Can you work these out from the model? Positions are in its coordinate system, mm. A direction names the side the tool comes from. Round coordinates to 2 decimals unless told otherwise and drop trailing zeros. Loops run counter-clockwise (first coordinate to the right, second up) from the corner with the lowest first, then second, coordinate; pieces in that order, holes last. Notation, with made-up numbers: (-11.75, 83) -> (22.25, 83) arc R24 cw to (22.25, 104) -> close; hole circle Ø6 at (-29.75, 7.5). An arc over 180 degrees is marked (long way). Use a Markdown table: item, result.
from build123d import *

# Parameters (mm, degrees)
CYLINDER_R        = 12.5
CYLINDER_DEPTH    = 4
CYLINDER001_R     = 11
CYLINDER001_DEPTH = 4
CYLINDER002_W     = 11
CYLINDER002_H     = 4
CYLINDER002_ANGLE = 66
BOX_W             = 5
BOX_H             = 1.9
BOX_DEPTH         = 4
BOX001_W          = 5
BOX001_H          = 1.9
BOX001_DEPTH      = 4
CYLINDER003_W     = 13
CYLINDER003_H     = 4
CYLINDER003_ANGLE = 60
CYLINDER004_W     = 14.25
CYLINDER004_H     = 4
CYLINDER004_ANGLE = 46
CYLINDER005_W     = 13
CYLINDER005_H     = 4
CYLINDER005_ANGLE = 60
CYLINDER006_W     = 14.25
CYLINDER006_H     = 4
CYLINDER006_ANGLE = 46
FILLET_R          = 0.9
FILLET001_R       = 0.6
FILLET002_R       = 1.2


with BuildPart() as part:
    # Cylinder → Cylinder (join)
    with BuildSketch(Plane.XY):
        Circle(CYLINDER_R)
    extrude(amount=CYLINDER_DEPTH)

    # Cylinder001 → Cylinder001 (cut)
    with BuildSketch(Plane.XY):
        Circle(CYLINDER001_R)
    extrude(amount=CYLINDER001_DEPTH, mode=Mode.SUBTRACT)

    # Cylinder002 → Cylinder002 (revolve, cut)
    with BuildSketch(Plane(origin=(0, 2, 0), x_dir=(0.544639035, 0.8386705679, 0), z_dir=(0.8386705679, -0.544639035, 0))):
        with Locations((5.5, 2)):
            Rectangle(CYLINDER002_W, CYLINDER002_H)
    revolve(axis=Axis((0, 2, 0), (0, 0, 1)), revolution_arc=CYLINDER002_ANGLE, mode=Mode.SUBTRACT)

    # Box → Box (join)
    with BuildSketch(Plane(origin=(5.2, 10, 0), x_dir=(-0.544639035, -0.8386705679, 0), z_dir=(0, 0, 1))):
        with Locations((2.5, 0.95)):
            Rectangle(BOX_W, BOX_H)
    extrude(amount=BOX_DEPTH)

    # Box001 → Box001 (join)
    with BuildSketch(Plane(origin=(-6.811, 9, 0), x_dir=(0.544639035, -0.8386705679, 0), z_dir=(0, 0, 1))):
        with Locations((2.5, 0.95)):
            Rectangle(BOX001_W, BOX001_H)
    extrude(amount=BOX001_DEPTH)

    # Cylinder003 → Cylinder003 (revolve)
    with BuildSketch(Plane(origin=(17.65, -10, 0), x_dir=(-1, 0, 0), z_dir=(0, 1, 0))):
        with Locations((6.5, 2)):
            Rectangle(CYLINDER003_W, CYLINDER003_H)
    revolve(axis=Axis((17.65, -10, 0), (0, 0, 1)), revolution_arc=CYLINDER003_ANGLE)

    # Cylinder004 → Cylinder004 (revolve, cut)
    with BuildSketch(Plane(origin=(21.75, -10, 0), x_dir=(-1, 0, 0), z_dir=(0, 1, 0))):
        with Locations((7.125, 2)):
            Rectangle(CYLINDER004_W, CYLINDER004_H)
    revolve(axis=Axis((21.75, -10, 0), (0, 0, 1)), revolution_arc=CYLINDER004_ANGLE, mode=Mode.SUBTRACT)

    # Cylinder005 → Cylinder005 (revolve)
    with BuildSketch(Plane(origin=(-17.6, -10, 0), x_dir=(0.5, -0.8660254038, 0), z_dir=(-0.8660254038, -0.5, 0))):
        with Locations((6.5, 2)):
            Rectangle(CYLINDER005_W, CYLINDER005_H)
    revolve(axis=Axis((-17.6, -10, 0), (0, 0, 1)), revolution_arc=CYLINDER005_ANGLE)

    # Cylinder006 → Cylinder006 (revolve, cut)
    with BuildSketch(Plane(origin=(-21.75, -10, 0), x_dir=(0.6946583705, -0.7193398003, 0), z_dir=(-0.7193398003, -0.6946583705, 0))):
        with Locations((7.125, 2)):
            Rectangle(CYLINDER006_W, CYLINDER006_H)
    revolve(axis=Axis((-21.75, -10, 0), (0, 0, 1)), revolution_arc=CYLINDER006_ANGLE, mode=Mode.SUBTRACT)

    # Fillet
    fillet_edges = [part.edges().sort_by_distance(p)[0] for p in [
        (-4.087805, 4.806647, 2),
        (-2.494331, 5.841461, 2),
        (4.070279, 4.771833, 2),
        (2.476805, 5.806647, 2),
    ]]
    fillet(fillet_edges, radius=FILLET_R)

    # Fillet001
    fillet001_edges = [part.edges().sort_by_distance(p)[0] for p in [
        (11.15, -21.25833, 2),
        (11.774728, -20.176269, 2),
        (-11.742835, -20.144907, 2),
        (-11.1, -21.25833, 2),
    ]]
    fillet(fillet001_edges, radius=FILLET001_R)

    # Fillet002
    fillet002_edges = [part.edges().sort_by_distance(p)[0] for p in [
        (-5.868544, 11.036765, 2),
        (5.868544, 11.036765, 2),
    ]]
    fillet(fillet002_edges, radius=FILLET002_R)


solid = part.part
1. Will this pin go through, and if not, where does the flat tip stop? pin 1 Ø2 at (x, y) = (-9.5, 0) entering from -Z.
Answer sheet:
| item | result |
|---|---|
| pin 1 | passes through |
2. I want a section at A-A (y = -2.5). Please give me the cut outline in (x, z).
Answer sheet:
| item | result |
|---|---|
| outline | (-12.25, 0) -> (-10.71, 0) -> (-10.71, 4) -> (-12.25, 4) -> close; (10.71, 0) -> (12.25, 0) -> (12.25, 4) -> (10.71, 4) -> close |
3. I want a section at C-C (y = -9). Please give me the cut outline in (x, z).
Answer sheet:
| item | result |
|---|---|
| outline | (-8.67, 0) -> (-6.32, 0) -> (-6.32, 4) -> (-8.67, 4) -> close; (6.32, 0) -> (8.67, 0) -> (8.67, 4) -> (6.32, 4) -> close |
4. I need wall thicknesses on line 1 (X direction, y = 8, z = 3.8); line 2 (X direction, y = 0, z = 2.25); line 3 (Y direction, x = 7.25, z = 1.4). Which ranges of each line are inside material? Lowest first, please.
Answer sheet:
| item | result |
|---|---|
| line 1 | x = -9.6 to -7.55, -6.16 to -3.9, 3.9 to 6.17, 7.55 to 9.6 |
| line 2 | x = -12.5 to -11, 11 to 12.5 |
| line 3 | y = -17.8 to -8.27, 8.27 to 10.18 |
5. If we mould it in two halves opening along Y, with no side actions, what happens to faces 4 (the cylindrical face through (-8.547, -15.362, 2.028)), 5 (the cylindrical face through (0, -11, 2)), 6 (the cylindrical face through (-11.02, -21.01, 2.03)), 7 (the flat face through (-4.117, 8.34, 1.972))? For each: +Y half, -Y half, draft (parallel to the pull), parting line (faces both ways), or undercut.
Answer sheet:
| item | result |
|---|---|
| face 4 | undercut |
| face 5 | undercut |
| face 6 | -Y half |
| face 7 | +Y half |
6. I want a section at D-D (x = 0). Please give me the cut outline in (y, z), plus the area to 3 significant figures.
Answer sheet:
| item | result |
|---|---|
| outline | (-12.5, 0) -> (-11, 0) -> (-11, 4) -> (-12.5, 4) -> close |
| area | 6.00 mm² |
7. Which directions (+Z, -Z, +X, -X, +Y, -Y) give clear straight access to the entire face, cutting with the end or side of a thin tool? Please do faces 1 (the cylindrical face through (6.59, -16.83, 2.03)), 2 (the flat face through (4.024, 8.189, 1.972)), 3 (the cylindrical face through (3.983, 5.134, 2.028)).
Answer sheet:
| item | result |
|---|---|
| face 1 | +Z, -Z, -Y |
| face 2 | +Z, -Z, +Y |
| face 3 | +Z, -Z |
